from build123d import *

# Parameters (mm, degrees)
SKETCH_1_R          = 38
EXTRUDE_1_DEPTH     = 3
SKETCH_2_R          = 16
CUT_EXTRUDE_2_DEPTH = 0.02
CUT_EXTRUDE_3_DEPTH = 0.1


with BuildPart() as part:
    # Эскиз1 → Вытянуть1 (new body)
    with BuildSketch(Plane.XY):
        with Locations((1.155432358, 0.834536784)):
            Circle(SKETCH_1_R)
    extrude(amount=EXTRUDE_1_DEPTH)

    # Эскиз2 → Вытянуть2 (cut)
    with BuildSketch(Plane.XY.offset(3)):
        Circle(SKETCH_2_R)
    extrude(amount=-CUT_EXTRUDE_2_DEPTH, mode=Mode.SUBTRACT)

    # Эскиз3 → Вытянуть3 (cut)
    # profile 1 of 3: a face of its own
    with BuildSketch(Plane.XY.offset(2.98)):
        with BuildLine():
            ThreePointArc((9.393894737, 2.302891329), (9.203408238, 2.705588354), (9.606105263, 2.896074853))
            ThreePointArc((9.606105263, 2.896074853), (9.870539579, 2.764896264), (10.097373549, 2.576005609))
            ThreePointArc((10.097373549, 2.576005609), (11.775195787, 3.127662368), (12.815, 1.7))
            Line((12.815, 1.7), (12.815, -1.485))
            ThreePointArc((12.815, -1.485), (12.5, -1.8), (12.185, -1.485))
            Line((12.185, -1.485), (12.185, 1.7))
            ThreePointArc((12.185, 1.7), (11.315, 2.57), (10.445, 1.7))
            Line((10.445, 1.7), (10.445, -1.485))
            ThreePointArc((10.445, -1.485), (10.13, -1.8), (9.815, -1.485))
            Line((9.815, -1.485), (9.815, 1.7))
            Line((9.815, 1.7), (9.815, 1.705))
            ThreePointArc((9.815, 1.705), (9.699157085, 2.070651365), (9.393894737, 2.302891329))
        make_face()
    # profile 2 of 3: a face of its own
    with BuildSketch(Plane.XY.offset(2.98)):
        with BuildLine():
            Line((-10.497591493, 1.756383955), (-10.635054332, 2.196407461))
            ThreePointArc((-10.635054332, 2.196407461), (-11.152905752, 2.922098665), (-12, 3.2))
            ThreePointArc((-12, 3.2), (-13.767766953, 2.467766953), (-14.5, 0.7))
            ThreePointArc((-14.5, 0.7), (-13.767766953, -1.067766953), (-12, -1.8))
            ThreePointArc((-12, -1.8), (-11.152905752, -1.522098665), (-10.635054332, -0.796407461))
            Line((-10.635054332, -0.796407461), (-10.497591493, -0.356383955))
            Line((-10.497591493, -0.356383955), (-10.11566985, -1.578928916))
            ThreePointArc((-10.11566985, -1.578928916), (-9.721071084, -1.78566985), (-9.51433015, -1.391071084))
            Line((-9.51433015, -1.391071084), (-10.167578358, 0.7))
            Line((-10.167578358, 0.7), (-9.51433015, 2.791071084))
            ThreePointArc((-9.51433015, 2.791071084), (-9.721071084, 3.18566985), (-10.11566985, 2.978928916))
            Line((-10.11566985, 2.978928916), (-10.497591493, 1.756383955))
        make_face()
        with BuildLine():
            Line((-10.827604629, 0.7), (-11.237145368, -0.610954683))
            ThreePointArc((-11.237145368, -0.610954683), (-11.527689249, -1.01570067), (-12.001425757, -1.170001613))
            ThreePointArc((-12.001425757, -1.170001613), (-13.32305175, -0.621529891), (-13.87000042, 0.700727136))
            ThreePointArc((-13.87000042, 0.700727136), (-13.322537782, 2.02204425), (-12.001425757, 2.570001613))
            ThreePointArc((-12.001425757, 2.570001613), (-11.527689249, 2.41570067), (-11.237145368, 2.010954683))
            Line((-11.237145368, 2.010954683), (-10.827604629, 0.7))
        make_face(mode=Mode.SUBTRACT)
    # profile 3 of 3: a face of its own
    with BuildSketch(Plane.XY.offset(2.98)):
        with BuildLine():
            ThreePointArc((14.515, -2.55), (14.420756237, -2.825567596), (14.1775, -2.985710626))
            ThreePointArc((14.1775, -2.985710626), (14.069763125, -3.168447502), (14.2525, -3.276184377))
            ThreePointArc((14.2525, -3.276184377), (14.657927061, -3.009279327), (14.815, -2.55))
            Line((14.815, -2.55), (14.815, 0.55))
            ThreePointArc((14.815, 0.55), (14.665, 0.7), (14.515, 0.55))
            Line((14.515, 0.55), (14.515, -1.05))
            ThreePointArc((14.515, -1.05), (14.065, -1.5), (13.615, -1.05))
            Line((13.615, -1.05), (13.615, 0.55))
            ThreePointArc((13.615, 0.55), (13.465, 0.7), (13.315, 0.55))
            Line((13.315, 0.55), (13.315, -1.05))
            ThreePointArc((13.315, -1.05), (13.729589803, -1.720820393), (14.515, -1.65))
            Line((14.515, -1.65), (14.515, -2.55))
        make_face()
    extrude(amount=-CUT_EXTRUDE_3_DEPTH, mode=Mode.SUBTRACT)


solid = part.part
Could you check a few things on this model? Use its own coordinates, in mm. A direction names the side the tool comes from. Give positions to 0.01 mm unless a question says otherwise; leave off trailing zeros. Order: outer loops, then holes, each group sorted by start corner. A loop starts at its lowest first (then second) coordinate and runs counter-clockwise, first axis right, second up.
1. For faces 4 (the flat face through (1, 1, 0)), 5 (the flat face through (10, 1, 2.88)), which set-ups out of +Z, -Z, +X, -X, +Y, -Y let a thin tool reach every point of the face, with its end or its side?
2. Suppose I cut it at D-D (y = 17). List the corners of the cut face in (x, z) for me, plus the area to 3 significant figures.
3. I need wall thicknesses on L1, parallel to Z at x = -7, y = -2; L2, parallel to Y at x = 2, z = 1.05; L3, parallel to X at y = 19, z = 2.35. Which ranges of each line are inside material? Lowest first, please.
4. Suppose I cut it at B-B (z = 1.15). List the corners of the cut face in (x, y) for me, plus the area to 3 significant figures.
5. Suppose I cut it at C-C (x = -19.5). List the corners of the cut face in (y, z) for me.
6. Will these pins go through, and if not, where does the flat tip stop? P1, Ø4, axis at x = -13, y = 0.5, coming from the +Z side; P2, Ø1.5, axis at x = -12.5, z = 2.5, coming from the +Y side; P3, Ø1, axis at x = -6, z = 1, coming from the -Y side.
7. We'd pull the mould along Y, two halves only. Please class faces 1 (the flat face through (18, 1, 3)), 2 (the cylindrical face through (21.58, 32.88, 1.48)), 3 (the flat face through (-11, 2, 2.88)): pulls with the +Y half, pulls with the -Y half, needs draft (parallel to the pull), parting line crosses it, or undercut.
Solved:
1. face 4: -Z, +X, -X, +Y, -Y
1. face 5: +Z
2. outline: (-33.23, 0) - (35.55, 0) - (35.55, 3) - (-33.23, 3) - close
2. area: 206 mm2
3. L1: z = 0 to 2.98
3. L2: y = -37.16 to 38.83
3. L3: x = -32.22 to 34.53
4. outline: circle Ø76 at (1.16, 0.83)
4. area: 4,540 mm2
5. outline: (-31.06, 0) - (32.73, 0) - (32.73, 3) - (-31.06, 3) - close
6. P1: stops at z = 2.98
6. P2: stops at y = 36.58
6. P3: stops at y = -36.58
7. face 1: needs draft
7. face 2: parting line crosses it
7. face 3: undercut
